from build123d import *

# Parameters (mm, degrees)
SKETCH2_R           = 1.5
BOSS_EXTRUDE1_DEPTH = 7
SKETCH4_OUTSIDE_W   = 6.638
SKETCH4_OUTSIDE_H   = 6.638
SKETCH4_OUTSIDE_R   = 0.9
CUT_EXTRUDE1_DEPTH  = 5.8
SKETCH5_OUTSIDE_W   = 6.638
SKETCH5_OUTSIDE_H   = 6.638
SKETCH5_OUTSIDE_R   = 0.85
CUT_EXTRUDE2_DEPTH  = 3.8
SKETCH6_W           = 3.2
SKETCH6_H           = 0.4
CUT_EXTRUDE3_DEPTH  = 0.5
CHAMFER1_SIZE       = 0.3


with BuildPart() as part:
    # Sketch2 → Boss-Extrude1 (new body)
    with BuildSketch(Plane.XY):
        Circle(SKETCH2_R)
    extrude(amount=-BOSS_EXTRUDE1_DEPTH)

    # Sketch4 outside → Cut-Extrude1 (cut)
    with BuildSketch(Plane(origin=(0, 0, -7), x_dir=(-1, 0, 0), z_dir=(0, 0, -1))):
        Rectangle(SKETCH4_OUTSIDE_W, SKETCH4_OUTSIDE_H)
        Circle(SKETCH4_OUTSIDE_R, mode=Mode.SUBTRACT)
    extrude(amount=-CUT_EXTRUDE1_DEPTH, mode=Mode.SUBTRACT)

    # Sketch5 outside → Cut-Extrude2 (cut)
    with BuildSketch(Plane(origin=(0, 0, -7), x_dir=(-1, 0, 0), z_dir=(0, 0, -1))):
        Rectangle(SKETCH5_OUTSIDE_W, SKETCH5_OUTSIDE_H)
        Circle(SKETCH5_OUTSIDE_R, mode=Mode.SUBTRACT)
    extrude(amount=-CUT_EXTRUDE2_DEPTH, mode=Mode.SUBTRACT)

    # Sketch6 → Cut-Extrude3 (cut)
    with BuildSketch(Plane.XY):
        Rectangle(SKETCH6_W, SKETCH6_H)
    extrude(amount=-CUT_EXTRUDE3_DEPTH, mode=Mode.SUBTRACT)

    # Chamfer1
    chamfer1_edges = [part.edges().sort_by_distance(p)[0] for p in [
        (0.85, 0, -7),
    ]]
    chamfer(chamfer1_edges, length=CHAMFER1_SIZE)


solid = part.part
Read the model definition and answer for the solid it produces. Units are mm, in the model's axes. A direction names the side the tool comes from. Give positions to 0.01 mm unless a question says otherwise; leave off trailing zeros. Loops run counter-clockwise (first coordinate to the right, second up) from the corner with the lowest first, then second, coordinate; pieces in that order, holes last. Notation, with made-up numbers: (-27, -39) -> (-18, -39) arc R3 ccw to (-18, -35) -> close; hole circle Ø9 at (55, 80). An arc over 180 degrees is marked (long way). Use a Markdown table: item, result.
Q1. Section A-A, the plane y = 0 is taken. Determine the outline of the cut face in (x, z).
Solved:
| item | result |
|---|---|
| outline | (-1.5, -1.2) -> (-0.9, -1.2) -> (-0.9, -3.2) -> (-0.85, -3.2) -> (-0.85, -6.7) -> (-0.55, -7) -> (0.55, -7) -> (0.85, -6.7) -> (0.85, -3.2) -> (0.9, -3.2) -> (0.9, -1.2) -> (1.5, -1.2) -> (1.5, -0.5) -> (-1.5, -0.5) -> close |
Q2. Determine the mould class of faces 3 (the face through (0, -1, 0)), 4 (the face through (-0.86, 0.27, -2.21)) for opening direction X: pulls with the +X half, pulls with the -X half, needs draft (parallel to the pull), parting line crosses it, or undercut.
Solved:
| item | result |
|---|---|
| face 3 | needs draft |
| face 4 | parting line crosses it |
Q3. Section D-D, the plane z = -1 is taken. Determine the outline of the cut face in (x, y), then the cut area to 3 significant figures.
Solved:
| item | result |
|---|---|
| outline | circle Ø3 at (0, 0) |
| area | 7.07 mm^2 |
Q4. Section B-B, the plane x = 0 is taken. Determine the outline of the cut face in (y, z).
Solved:
| item | result |
|---|---|
| outline | (-1.5, -1.2) -> (-0.9, -1.2) -> (-0.9, -3.2) -> (-0.85, -3.2) -> (-0.85, -6.7) -> (-0.55, -7) -> (0.55, -7) -> (0.85, -6.7) -> (0.85, -3.2) -> (0.9, -3.2) -> (0.9, -1.2) -> (1.5, -1.2) -> (1.5, 0) -> (0.2, 0) -> (0.2, -0.5) -> (-0.2, -0.5) -> (-0.2, 0) -> (-1.5, 0) -> close |
Q5. Section C-C, the plane z = -3.75 is taken. Determine the outline of the cut face in (x, y), then the cut area to 3 significant figures.
Solved:
| item | result |
|---|---|
| outline | circle Ø1.7 at (0, 0) |
| area | 2.27 mm^2 |
Q6. Each of these flat-tipped pins is pushed along its axis until it touches: pin 1 (0.9 mm diameter, centred on x = 0.5, y = -0.5, fed in from -Z); pin 2 (1.5 mm diameter, centred on x = 0, z = -5, fed in from -Y); pin 3 (1 mm diameter, centred on y = -0.5, z = -4.5, fed in from +X). Where does it stop, or does it pass through?
Solved:
| item | result |
|---|---|
| pin 1 | stops at z = -7 |
| pin 2 | stops at y = -0.85 |
| pin 3 | stops at x = 0.85 |
Q7. Find the intervals of material crossed by line 1 along Y through (x, z) = (0.3, -1.25); line 2 along Z through (x, y) = (-1, 0.55); line 3 along Y through (x, z) = (1.3, -0.25), in increasing order.
Solved:
| item | result |
|---|---|
| line 1 | y = -0.85 to 0.85 |
| line 2 | z = -1.2 to 0 |
| line 3 | y = -0.75 to -0.2, 0.2 to 0.75 |
Q8. A tool of negligible diameter and unlimited length cuts with its end or side. For faces 1 (the face through (0, 0, -7)), 2 (the face through (0.18, -0.83, -4.97)), from which of +Z, -Z, +X, -X, +Y, -Y can it reach the whole face along a straight path? Write none if from no direction.
Solved:
| item | result |
|---|---|
| face 1 | -Z, +X, -X, +Y, -Y |
| face 2 | -Z |
